```python
from build123d import *

# Parameters (mm, degrees)
F1_DEPTH = 114.3
F2_DEPTH = 114.3


with BuildPart() as f1:
    # F0 (on Right) → F1 (new body)
    with BuildSketch(Plane.YZ):
        with BuildLine():
            ThreePointArc((15.3397259396, 4.9735903311), (33.2535851209, 2.1483766452), (50.5945171187, 7.4568849653))
            Line((50.5945171187, 7.4568849653), (62.121764605, -1.4823092679))
            Line((62.121764605, -1.4823092679), (65.296764605, -1.4823092679))
            Line((65.296764605, -1.4823092679), (65.296764605, 17.0836517627))
            Line((65.296764605, 17.0836517627), (-74.4234208748, 17.0836517627))
            Line((-74.4234208748, 17.0836517627), (-74.4234208748, 8.8286517627))
            Line((-74.4234208748, 8.8286517627), (-55.3734208748, 8.8286517627))
            Line((-55.3734208748, 8.8286517627), (-55.3734208748, 0.8911517627))
            Line((-55.3734208748, 0.8911517627), (-49.1014425221, 8.0960725076))
            ThreePointArc((-49.1014425221, 8.0960725076), (-48.7232814382, 8.2705023504), (-48.3417610399, 8.1035479821))
            ThreePointArc((-48.3417610399, 8.1035479821), (-36.4490241706, 2.7123313027), (-24.3859868745, 7.7108849653))
            Line((-24.3859868745, 7.7108849653), (-18.6202428219, 3.4182849653))
            ThreePointArc((-18.6202428219, 3.4182849653), (-7.7779010166, 8.4768928848), (4.1840897409, 8.2388445204))
            ThreePointArc((4.1840897409, 8.2388445204), (9.8069500348, 6.7601026388), (15.3397259396, 4.9735903311))
        make_face()
    extrude(amount=F1_DEPTH)

    # F2 (add): a face of the model
    f2_faces = [f1.faces().sort_by_distance(p)[0] for p in [
        (0, 0.4923148954, 10.8715185192),
    ]]
    extrude(f2_faces, amount=F2_DEPTH)


solid = f1.part
```
For this review, take the finished solid that the model builds, in its own axes (mm). A direction names the side the tool comes from. Round coordinates to 2 decimals unless told otherwise and drop trailing zeros. Write each loop counter-clockwise with the first axis right and the second up, starting at its lowest first coordinate (ties: lowest second). Pieces come first, ordered by that corner, then holes. Notation, with made-up numbers: M -33.75,35.5 L -20.75,35.5 A14 ccw -20.75,49.5 Z; hole C 28.25,20.5 d6. An arc over 180 degrees is marked long. One line per item, written item: value. Start each with the question number.
(1) We need section B-B (y = -27.5). Give the boundary of the cut face in (x, z), and give its area (3 significant figures).
(2) We need section A-A (x = 46). Give the boundary of the cut face in (y, z).
(3) Machinability: for faces 1 (the flat face through (2, -55.373, 5)), 2 (the cylindrical face through (1.6, 9.729, 6.783)), 3 (the flat face through (2, 65.297, 8)), which of the approach directions +Z, -Z, +X, -X, +Y, -Y give a long, thin tool a straight path to every point of the face, cutting with its end or side? Answer none if there is none.
(4) Wall thickness on line 1 (Z direction, x = 87, y = -5.5); line 2 (Y direction, x = 49.5, z = 2); line 3 (Z direction, x = -91, y = -65): over which ranges is each line inside the solid? List them lowest first.
(5) We need section C-C (y = 12). Give the boundary of the cut face in (x, z).
(6) Insertion check: pin 1 (2 mm diameter, centred on x = 51, y = -41.5, fed in from -Z); pin 2 (5.5 mm diameter, centred on x = -19, y = -61, fed in from -Z); pin 3 (5 mm diameter, centred on x = -77.5, y = 7, fed in from -Z). Each pin has a flat end and moves straight along its axis. Give the tip position at first contact, or say it passes through.
(7) The part is to be moulded in two halves that separate along Y. For faces 4 (the flat face through (1.6, 56.28, 3.05)), 5 (the flat face through (2, -4, 17.084)), 6 (the cylindrical face through (1.6, -7.943, 8.441)), 7 (the flat face through (2, -74.423, 13)), say which applies: released by +Y, released by -Y, zero draft, split by the parting line, or undercut.
Result:
1. outline: M -114.3,5.19 L 114.3,5.19 L 114.3,17.08 L -114.3,17.08 Z
1. area: 2,720 mm²
2. outline: M -74.42,8.83 L -55.37,8.83 L -55.37,0.89 L -49.1,8.1 A0.51 cw -48.34,8.1 A16.41 ccw -24.39,7.71 L -18.62,3.42 A26.44 cw 4.18,8.24 A105.41 cw 15.34,4.97 A40.34 ccw 50.59,7.46 L 62.12,-1.48 L 65.3,-1.48 L 65.3,17.08 L -74.42,17.08 Z
3. face 1: -Z, +X, -X, -Y
3. face 2: -Z, +X, -X
3. face 3: +Z, -Z, +X, -X, +Y
4. line 1: 8.86 to 17.08
4. line 2: -55.37 to -54.41, 57.63 to 65.3
4. line 3: 8.83 to 17.08
5. outline: M -114.3,6.09 L 114.3,6.09 L 114.3,17.08 L -114.3,17.08 Z
6. pin 1: z = 3.29
6. pin 2: z = 8.83
6. pin 3: z = 6.85
7. face 4: undercut
7. face 5: zero draft
7. face 6: undercut
7. face 7: released by -Y
